Geometry: final body of the model. Coordinates: model frame, mm. Face numbers are marked on the shaded views. Give positions to 0.01 mm unless a question says otherwise; leave off trailing zeros. Write each loop counter-clockwise with the first axis right and the second up, starting at its lowest first coordinate (ties: lowest second). Pieces come first, ordered by that corner, then holes.
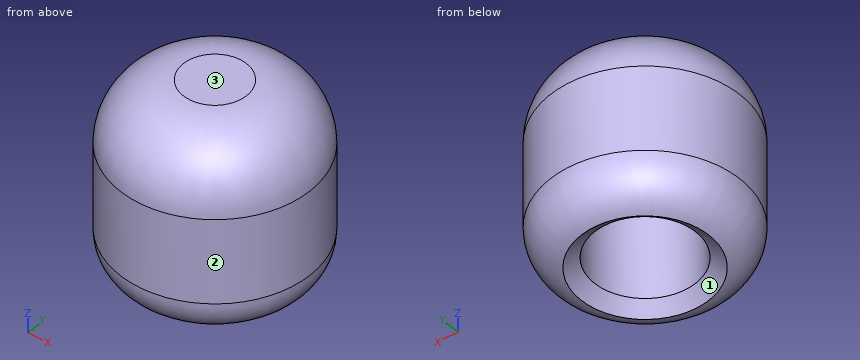
from build123d import *

# Parameters (mm, degrees)
SKETCH1_R           = 4.5
SKETCH1_R_2         = 2.4
BOSS_EXTRUDE1_DEPTH = 9
FILLET1_R           = 3
FILLET2_R           = 2
SKETCH1_4_R         = 2.4
CUT_EXTRUDE2_DEPTH  = 6


with BuildPart() as part:
    # Sketch1 → Boss-Extrude1 (new body)
    # profile 1 of 2: a face of its own
    with BuildSketch(Plane.XY):
        Circle(SKETCH1_R)
        Circle(SKETCH1_R_2, mode=Mode.SUBTRACT)
    # profile 2 of 2: a face of its own
    with BuildSketch(Plane.XY):
        Circle(SKETCH1_R_2)
    extrude(amount=BOSS_EXTRUDE1_DEPTH)

    # Fillet1
    fillet1_edges = [part.edges().sort_by_distance(p)[0] for p in [
        (-4.5, 0, 9),
    ]]
    fillet(fillet1_edges, radius=FILLET1_R)

    # Fillet2
    fillet2_edges = [part.edges().sort_by_distance(p)[0] for p in [
        (-4.5, 0, 0),
    ]]
    fillet(fillet2_edges, radius=FILLET2_R)

    # Sketch1<4> → Cut-Extrude2 (cut, symmetric)
    with BuildSketch(Plane.XY):
        Circle(SKETCH1_4_R)
    extrude(amount=CUT_EXTRUDE2_DEPTH, both=True, mode=Mode.SUBTRACT)

    # Chamfer1: read off the stored shape, not the designer's step
    # Chamfer1 outline → Chamfer1 (revolve, cut)
    with BuildSketch(Plane.XZ):
        Polygon((2.4, 0.554316771), (2.4, 0), (3.033333333, 0), (3.033333333, 0.072422361), align=None)
    revolve(axis=Axis((0, 0, 0), (0, 0, 1)), mode=Mode.SUBTRACT)


solid = part.part
Q1. Ray query, line 1 along Y through (x, z) = (0, 4.7); line 2 along Y through (x, z) = (0.5, 2); line 3 along X through (y, z) = (1.5, 1). Return the intervals inside material, ascending.
Filled sheet:
line 1: y = -4.5 to -2.4, 2.4 to 4.5
line 2: y = -4.47 to -2.35, 2.35 to 4.47
line 3: x = -3.96 to -1.87, 1.87 to 3.96
Q2. Pull-direction query (Y, two-part tool) for the marked faces 1, 2 and 3; classes: released by +Y, released by -Y, zero draft, split by the parting line, or undercut.
Filled sheet:
face 1: undercut
face 2: split by the parting line
face 3: zero draft
Q3. Section B-B on z = 1.75. Output: boundary loops of the cut face in (x, y).
Filled sheet:
outline: circle Ø8.97 at (0, 0); hole circle Ø4.8 at (0, 0)
Q4. Pin query (flat end, axial travel): P1, Ø3, axis at x = 2.5, z = 1, coming from the +Y side; P2, Ø1, axis at x = -2, y = -1, coming from the -Z side; P3, Ø4, axis at y = 2.5, z = 5, coming from the +X side. Return the tip coordinate at first contact, or that it passes through.
Filled sheet:
P1: stops at y = 4.32
P2: stops at z = 0.3
P3: stops at x = 4.47
Q5. Section A-A on z = 2.75. Output: boundary loops of the cut face in (x, y), plus the area to 3 significant figures.
Filled sheet:
outline: circle Ø9 at (0, 0); hole circle Ø4.8 at (0, 0)
area: 45.5 mm2
